Input: part model. Units: mm. Frame: model coordinates. A direction names the side the tool comes from. Give positions to 0.01 mm unless a question says otherwise; leave off trailing zeros. Loops run counter-clockwise (first coordinate to the right, second up) from the corner with the lowest first, then second, coordinate; pieces in that order, holes last. Notation, with made-up numbers: M 57.5,-23 L 114.5,-23 A21 ccw 114.5,15 Z; hole C 31.5,19 d6. An arc over 180 degrees is marked long. Answer as a JSON object with one key per item and string values. Group by question number.
1) Section query A-A on x = -3. Return loops of the section in (y, z), plus the area to 3 significant figures.
2) Ray query, L1, parallel to Z at x = 1.5, y = 1.5; L2, parallel to Z at x = -8.5, y = -0.5; L3, parallel to Y at x = -1, z = -2.5. Return the intervals inside material, ascending.
3) Draft query along Y for faces 1 (the flat face through (-5, -2, -6)), 2 (the flat face through (-4, 15.92, -5)), 3 (the cylindrical face through (-0.33, 13.53, 2.48)), 4 (the cylindrical face through (-9.224, -2.052, -2.958)). Return one class per face: +Y half, -Y half, draft (parallel to the pull), parting line (faces both ways), or undercut.
4) Access query for faces 5 (the flat face through (-5, 14.802, 2)), 6 (the flat face through (-5, -3.377, -3)), 7 (the cylindrical face through (-0.33, -2.11, 1.25)). Directions: +Z, -Z, +X, -X, +Y, -Y. A direction counts if a zero-diameter tool reaches every point of the face in a straight line with its end or side. Return the directions, or none.
5) First-contact query: P1, Ø3, axis at x = -3.5, y = 13, coming from the +Z side; P2, Ø2.5, axis at x = -5, z = 2.5, coming from the -Y side; P3, Ø2, axis at x = -5.5, y = -1.5, coming from the -Z side. Flat tips, straight axial feed; report the tip coordinate or a pass-through.
6) Section query C-C on z = 7.75. Return loops of the section in (x, y).
7) Section query B-B on y = 9. Return loops of the section in (x, z) (3 decimals), plus the area to 3 significant figures.
8) Section query D-D on x = -18.5. Return loops of the section in (y, z), plus the area to 3 significant figures.
from build123d import *

# Parameters (mm, degrees)
ESQUISSE1_W             = 45
ESQUISSE1_H             = 20
BOSS_EXTRU_1_DEPTH      = 1
ESQUISSE2_R             = 9
BOSS_EXTRU_3_DEPTH      = 14
BOSS_EXTRU_4_DEPTH      = 3
BOSS_EXTRU_5_DEPTH      = 6
BOSS_EXTRU_5_DEPTH_BACK = 1.5
SKETCH3_W               = 45
SKETCH3_H               = 10
BOSS_EXTRUDE1_DEPTH     = 12
CHAMFER1_SIZE           = 11


with BuildPart() as part:
    # Esquisse1 → Boss.-Extru.1 (new body)
    with BuildSketch(Plane.XY):
        with Locations((-4.778042712, 5.919811321)):
            Rectangle(ESQUISSE1_W, ESQUISSE1_H)
    extrude(amount=BOSS_EXTRU_1_DEPTH)

    # Esquisse2 → Boss.-Extru.3 (add)
    with BuildSketch(Plane.XY.offset(1)):
        with Locations((-17.828042712, 5.456465128)):
            Circle(ESQUISSE2_R)
        with Locations((8.271957288, 5.410130508)):
            Circle(ESQUISSE2_R)
    extrude(amount=BOSS_EXTRU_3_DEPTH)

    # Esquisse3 → Boss.-Extru.4 (add)
    with BuildSketch(Plane.XY.offset(1)):
        with BuildLine():
            Line((-7.928796825, 14.80247516), (-1.627288599, 14.80247516))
            ThreePointArc((-1.627288599, 14.80247516), (-0.329919258, 13.505105819), (-1.627288599, 12.207736479))
            Line((-1.627288599, 12.207736479), (-7.928796825, 12.207736479))
            ThreePointArc((-7.928796825, 12.207736479), (-9.226166166, 13.505105819), (-7.928796825, 14.80247516))
        make_face()
    extrude(amount=BOSS_EXTRU_4_DEPTH)

    # Esquisse4 → Boss.-Extru.5 (add, two sides: drawn at the far end of the back side and taken through both)
    with BuildSketch(Plane(origin=(0.9463019, -1.208788393, 0), x_dir=(-1, 0, 0), z_dir=(0, 0, -1)).offset(-BOSS_EXTRU_5_DEPTH_BACK)):
        with BuildLine():
            Line((2.572836386, 0.424993111), (8.874344612, 0.424993111))
            ThreePointArc((8.874344612, 0.424993111), (10.17073801, -0.871400286), (8.874344612, -2.167793683))
            Line((8.874344612, -2.167793683), (2.572836386, -2.167793683))
            ThreePointArc((2.572836386, -2.167793683), (1.276442989, -0.871400286), (2.572836386, 0.424993111))
        make_face()
    extrude(amount=BOSS_EXTRU_5_DEPTH + BOSS_EXTRU_5_DEPTH_BACK)

    # Sketch3 → Boss-Extrude1 (add)
    with BuildSketch(Plane(origin=(0, 0, 0), x_dir=(-1, 0, 0), z_dir=(0, 0, -1))):
        with Locations((4.778042712, 10.919811321)):
            Rectangle(SKETCH3_W, SKETCH3_H)
    extrude(amount=BOSS_EXTRUDE1_DEPTH)

    # Chamfer1
    # the kernel refuses this chamfer: 11 mm, written as the material it takes off along each edge
    with BuildSketch(Plane(origin=(-55.56655558, 5.919811321, -12), x_dir=(0, 0.9996219169112968, -0.027495876610586417), z_dir=(1, 0, 0))) as chamfer1_piece_1:
        Polygon((CHAMFER1_SIZE * 0.999621916911, CHAMFER1_SIZE * 0.0274958766106), (-CHAMFER1_SIZE * 0.0274958766106, CHAMFER1_SIZE * 0.999621916911), (0, 0), align=None)
    extrude(amount=101.577025735, mode=Mode.SUBTRACT)


solid = part.part
Output:
{
 "1": {"outline": "M -4.08,0 L -3.38,0 L -3.38,-6 L -0.78,-6 L -0.78,0 L 5.92,0 L 5.92,-1 L 15.92,-11 L 15.92,1 L 14.8,1 L 14.8,4 L 12.21,4 L 12.21,1 L -0.78,1 L -0.78,1.5 L -3.38,1.5 L -3.38,1 L -4.08,1 Z", "area": "105 mm^2"},
 "2": {"L1": "z = 0 to 15", "L2": "z = 0 to 1", "L3": "y = -3.22 to -0.95, 7.42 to 15.92"},
 "3": {"face 1": "draft", "face 2": "+Y half", "face 3": "undercut", "face 4": "undercut"},
 "4": {"face 5": "+Z, +X, -X, +Y", "face 6": "-Z, +X, -X, -Y", "face 7": "+Z"},
 "5": {"P1": "stops at z = 4", "P2": "stops at y = -3.38", "P3": "stops at z = -6"},
 "6": {"outline": "C -17.83,5.46 d18; C 8.27,5.41 d18"},
 "7": {"outline": "M -27.278,-4.08 L 17.722,-4.08 L 17.722,1 L 16.525,1 L 16.525,15 L 0.019,15 L 0.019,1 L -9.555,1 L -9.555,15 L -26.101,15 L -26.101,1 L -27.278,1 Z", "area": "691 mm^2"},
 "8": {"outline": "M -4.08,0 L 5.92,0 L 5.92,-1 L 15.92,-11 L 15.92,1 L 14.43,1 L 14.43,15 L -3.52,15 L -3.52,1 L -4.08,1 Z", "area": "331 mm^2"}
}
